from build123d import *

# Parameters (mm, degrees)
SKETCH1_R           = 13
BOSS_EXTRUDE1_DEPTH = 20
SKETCH2_R           = 12.227815656
CUT_EXTRUDE1_DEPTH  = 14
SKETCH3_R           = 0.378353797
CUT_EXTRUDE2_DEPTH  = 0.3
FILLET1_R           = 0.5


with BuildPart() as part:
    # Sketch1 → Boss-Extrude1 (new body)
    with BuildSketch(Plane.XY):
        Circle(SKETCH1_R)
    extrude(amount=BOSS_EXTRUDE1_DEPTH)

    # Sketch2 → Cut-Extrude1 (cut)
    with BuildSketch(Plane.XY.offset(20)):
        Circle(SKETCH2_R)
    extrude(amount=-CUT_EXTRUDE1_DEPTH, mode=Mode.SUBTRACT)

    # Sketch3 → Cut-Extrude2 (cut)
    with BuildSketch(Plane.XY.offset(6)):
        with Locations((0, 10.077969325)):
            Circle(SKETCH3_R)
        with Locations((0, 8.577969325)):
            Circle(SKETCH3_R)
        with Locations((0, 7.077969325)):
            Circle(SKETCH3_R)
        with Locations((0, 5.577969325)):
            Circle(SKETCH3_R)
        with Locations((0, 4.077969325)):
            Circle(SKETCH3_R)
        with Locations((0, 2.577969325)):
            Circle(SKETCH3_R)
        with Locations((5.038984662, 8.727777454)):
            Circle(SKETCH3_R)
        with Locations((4.288984662, 7.428739348)):
            Circle(SKETCH3_R)
        with Locations((3.538984662, 6.129701243)):
            Circle(SKETCH3_R)
        with Locations((2.788984662, 4.830663137)):
            Circle(SKETCH3_R)
        with Locations((2.038984662, 3.531625031)):
            Circle(SKETCH3_R)
        with Locations((1.288984662, 2.232586926)):
            Circle(SKETCH3_R)
        with Locations((8.727777454, 5.038984662)):
            Circle(SKETCH3_R)
        with Locations((7.428739348, 4.288984662)):
            Circle(SKETCH3_R)
        with Locations((6.129701243, 3.538984662)):
            Circle(SKETCH3_R)
        with Locations((4.830663137, 2.788984662)):
            Circle(SKETCH3_R)
        with Locations((3.531625031, 2.038984662)):
            Circle(SKETCH3_R)
        with Locations((2.232586926, 1.288984662)):
            Circle(SKETCH3_R)
        with Locations((10.077969325, 0)):
            Circle(SKETCH3_R)
        with Locations((8.577969325, 0)):
            Circle(SKETCH3_R)
        with Locations((7.077969325, 0)):
            Circle(SKETCH3_R)
        with Locations((5.577969325, 0)):
            Circle(SKETCH3_R)
        with Locations((4.077969325, 0)):
            Circle(SKETCH3_R)
        with Locations((2.577969325, 0)):
            Circle(SKETCH3_R)
        with Locations((8.727777454, -5.038984662)):
            Circle(SKETCH3_R)
        with Locations((7.428739348, -4.288984662)):
            Circle(SKETCH3_R)
        with Locations((6.129701243, -3.538984662)):
            Circle(SKETCH3_R)
        with Locations((4.830663137, -2.788984662)):
            Circle(SKETCH3_R)
        with Locations((3.531625031, -2.038984662)):
            Circle(SKETCH3_R)
        with Locations((2.232586926, -1.288984662)):
            Circle(SKETCH3_R)
        with Locations((5.038984662, -8.727777454)):
            Circle(SKETCH3_R)
        with Locations((4.288984662, -7.428739348)):
            Circle(SKETCH3_R)
        with Locations((3.538984662, -6.129701243)):
            Circle(SKETCH3_R)
        with Locations((2.788984662, -4.830663137)):
            Circle(SKETCH3_R)
        with Locations((2.038984662, -3.531625031)):
            Circle(SKETCH3_R)
        with Locations((1.288984662, -2.232586926)):
            Circle(SKETCH3_R)
        with Locations((0, -10.077969325)):
            Circle(SKETCH3_R)
        with Locations((0, -8.577969325)):
            Circle(SKETCH3_R)
        with Locations((0, -7.077969325)):
            Circle(SKETCH3_R)
        with Locations((0, -5.577969325)):
            Circle(SKETCH3_R)
        with Locations((0, -4.077969325)):
            Circle(SKETCH3_R)
        with Locations((0, -2.577969325)):
            Circle(SKETCH3_R)
        with Locations((-5.038984662, -8.727777454)):
            Circle(SKETCH3_R)
        with Locations((-4.288984662, -7.428739348)):
            Circle(SKETCH3_R)
        with Locations((-3.538984662, -6.129701243)):
            Circle(SKETCH3_R)
        with Locations((-2.788984662, -4.830663137)):
            Circle(SKETCH3_R)
        with Locations((-2.038984662, -3.531625031)):
            Circle(SKETCH3_R)
        with Locations((-1.288984662, -2.232586926)):
            Circle(SKETCH3_R)
        with Locations((-8.727777454, -5.038984662)):
            Circle(SKETCH3_R)
        with Locations((-7.428739348, -4.288984662)):
            Circle(SKETCH3_R)
        with Locations((-6.129701243, -3.538984662)):
            Circle(SKETCH3_R)
        with Locations((-4.830663137, -2.788984662)):
            Circle(SKETCH3_R)
        with Locations((-3.531625031, -2.038984662)):
            Circle(SKETCH3_R)
        with Locations((-2.232586926, -1.288984662)):
            Circle(SKETCH3_R)
        with Locations((-10.077969325, 0)):
            Circle(SKETCH3_R)
        with Locations((-8.577969325, 0)):
            Circle(SKETCH3_R)
        with Locations((-7.077969325, 0)):
            Circle(SKETCH3_R)
        with Locations((-5.577969325, 0)):
            Circle(SKETCH3_R)
        with Locations((-4.077969325, 0)):
            Circle(SKETCH3_R)
        with Locations((-2.577969325, 0)):
            Circle(SKETCH3_R)
        with Locations((-8.727777454, 5.038984662)):
            Circle(SKETCH3_R)
        with Locations((-7.428739348, 4.288984662)):
            Circle(SKETCH3_R)
        with Locations((-6.129701243, 3.538984662)):
            Circle(SKETCH3_R)
        with Locations((-4.830663137, 2.788984662)):
            Circle(SKETCH3_R)
        with Locations((-3.531625031, 2.038984662)):
            Circle(SKETCH3_R)
        with Locations((-2.232586926, 1.288984662)):
            Circle(SKETCH3_R)
        with Locations((-5.038984662, 8.727777454)):
            Circle(SKETCH3_R)
        with Locations((-4.288984662, 7.428739348)):
            Circle(SKETCH3_R)
        with Locations((-3.538984662, 6.129701243)):
            Circle(SKETCH3_R)
        with Locations((-2.788984662, 4.830663137)):
            Circle(SKETCH3_R)
        with Locations((-2.038984662, 3.531625031)):
            Circle(SKETCH3_R)
        with Locations((-1.288984662, 2.232586926)):
            Circle(SKETCH3_R)
    extrude(amount=-CUT_EXTRUDE2_DEPTH, mode=Mode.SUBTRACT)

    # Fillet1
    fillet1_edges = [part.edges().sort_by_distance(p)[0] for p in [
        (-13, 0, 20),
    ]]
    fillet(fillet1_edges, radius=FILLET1_R)


solid = part.part
Geometry: final body of the model. Coordinates: model frame, mm. Give positions to 0.01 mm unless a question says otherwise; leave off trailing zeros. Write each loop counter-clockwise with the first axis right and the second up, starting at its lowest first coordinate (ties: lowest second). Pieces come first, ordered by that corner, then holes. Notation, with made-up numbers: (-11.75, 7.5) -> (29.25, 7.5) arc R28 ccw to (29.25, 41.5) -> close; hole circle Ø11 at (-27, 34.25). An arc over 180 degrees is marked (long way). Answer in a Markdown table with one row per item.
(1) Ray query, line 1 along X through (y, z) = (-8, 18.5); line 2 along Y through (x, z) = (8.5, 16.25); line 3 along Z through (x, y) = (-1.5, -4.25). Return the intervals inside material, ascending. Write a range as [from, to].
Answers below:
| item | result |
|---|---|
| line 1 | [-10.25, -9.25], [9.25, 10.25] |
| line 2 | [-9.84, -8.79], [8.79, 9.84] |
| line 3 | [0, 6] |
(2) Section query A-A on z = 8.75. Return loops of the section in (x, y), then the cut area to 3 significant figures.
Answers below:
| item | result |
|---|---|
| outline | circle Ø26 at (0, 0); hole circle Ø24.46 at (0, 0) |
| area | 61.2 mm^2 |
(3) Section query B-B on z = 4.25. Return loops of the section in (x, y), then the cut area to 3 significant figures.
Answers below:
| item | result |
|---|---|
| outline | circle Ø26 at (0, 0) |
| area | 531 mm^2 |
(4) Pin query (flat end, axial travel): pin 1 (1 mm diameter, centred on y = -2, z = 14, fed in from -X); pin 2 (1.5 mm diameter, centred on y = 3, z = 4.5, fed in from -X); pin 3 (0.8 mm diameter, centred on x = 8.5, y = -5, fed in from +Z). Return the tip coordinate at first contact, or that it passes through.
Answers below:
| item | result |
|---|---|
| pin 1 | x = -12.91 |
| pin 2 | x = -12.8 |
| pin 3 | z = 6 |
(5) Draft query along Y for faces 1 (the cylindrical face through (-10.316, -7.91, 9.614)), 2 (the cylindrical face through (11.663, 3.673, 13.098)), 3 (the flat face through (0, 0, 0)). Return one class per face: +Y half, -Y half, draft (parallel to the pull), parting line (faces both ways), or undercut.
Answers below:
| item | result |
|---|---|
| face 1 | parting line |
| face 2 | undercut |
| face 3 | draft |
